```python
from build123d import *

# Parameters (mm, degrees)
SKETCH_2_R      = 2
SKETCH_2_R_2    = 1
EXTRUDE_1_DEPTH = 5


with BuildPart() as part:
    # 草图2 → 凸台-拉伸1 (new body)
    # profile 1 of 3: a face of its own
    with BuildSketch(Plane.XY):
        Circle(SKETCH_2_R)
        Circle(SKETCH_2_R_2, mode=Mode.SUBTRACT)
    # profile 2 of 3: a face of its own
    with BuildSketch(Plane.XY):
        with BuildLine():
            ThreePointArc((2, 0), (1.414213562, -1.414213562), (0, -2))
            Line((0, -2), (80, -2))
            ThreePointArc((80, -2), (78, 0), (80, 2))
            Line((80, 2), (0, 2))
            ThreePointArc((0, 2), (1.414213562, 1.414213562), (2, 0))
        make_face()
    # profile 3 of 3: a face of its own
    with BuildSketch(Plane.XY):
        with Locations((80, 0)):
            Circle(SKETCH_2_R)
        with Locations((80, 0)):
            Circle(SKETCH_2_R_2, mode=Mode.SUBTRACT)
    extrude(amount=EXTRUDE_1_DEPTH)


solid = part.part
```
Verification items for the finished model (mm, model axes). Round coordinates to 2 decimals unless told otherwise and drop trailing zeros. Write each loop counter-clockwise with the first axis right and the second up, starting at its lowest first coordinate (ties: lowest second). Pieces come first, ordered by that corner, then holes. Notation, with made-up numbers: (86, 73.5) -> (126, 73.5) arc R25 cw to (126, 94.5) -> close; hole circle Ø11 at (-10.5, -17). An arc over 180 degrees is marked (long way). Write each question's results on one line, items separated by ' | '.
Q1. Thickness scan on probe 1 along Y at (x, z) = (80, 1.7); probe 2 along X at (y, z) = (0.6, 2.2); probe 3 along X at (y, z) = (-1.7, 1.65). Record the ranges inside material, lowest first.
Derived:
probe 1: y = -2 to -1, 1 to 2 | probe 2: x = -1.91 to -0.8, 0.8 to 79.2, 80.8 to 81.91 | probe 3: x = -1.05 to 81.05
Q2. Draft check along X on faces 1 (the face through (0, -1, 2)), 2 (the face through (39, -2, 2)), 3 (the face through (-2, 0, 2)), 4 (the face through (79, 0, 2)). Enter one of: released by +X, released by -X, zero draft, split by the parting line, or undercut.
Derived:
face 1: undercut | face 2: zero draft | face 3: released by -X | face 4: undercut
Q3. Go/stop test with a flat-tipped pin: pin 1 Ø1.6 at (x, y) = (80, 0) entering from +Z. Record where the tip stops, or that it passes through.
Derived:
pin 1: passes through
Q4. Sectioned sample at A-A, the plane y = 0. Record the boundary of the cut face in (x, z).
Derived:
outline: (-2, 0) -> (-1, 0) -> (-1, 5) -> (-2, 5) -> close; (1, 0) -> (79, 0) -> (79, 5) -> (1, 5) -> close; (81, 0) -> (82, 0) -> (82, 5) -> (81, 5) -> close
Q5. Sectioned sample at B-B, the plane z = 1.8. Record the boundary of the cut face in (x, y).
Derived:
outline: (0, -2) -> (80, -2) arc R2 ccw to (80, 2) -> (0, 2) arc R2 ccw to start; hole circle Ø2 at (0, 0); hole circle Ø2 at (80, 0)
